Job drawing, mm, ordinate dimensions from the low corner. One solid piece. Coordinates: 2 decimals unless noted, no trailing zeros. Write each loop counter-clockwise with the first axis right and the second up, starting at its lowest first coordinate (ties: lowest second). Pieces come first, ordered by that corner, then holes. Notation, with made-up numbers: (4.5, 22) - (59.5, 22) arc R5 cw to (59.5, 26) - close; hole circle Ø7 at (31, 18.25). An arc over 180 degrees is marked (long way). Use one line per item in the form item = value. Start each with the question number.
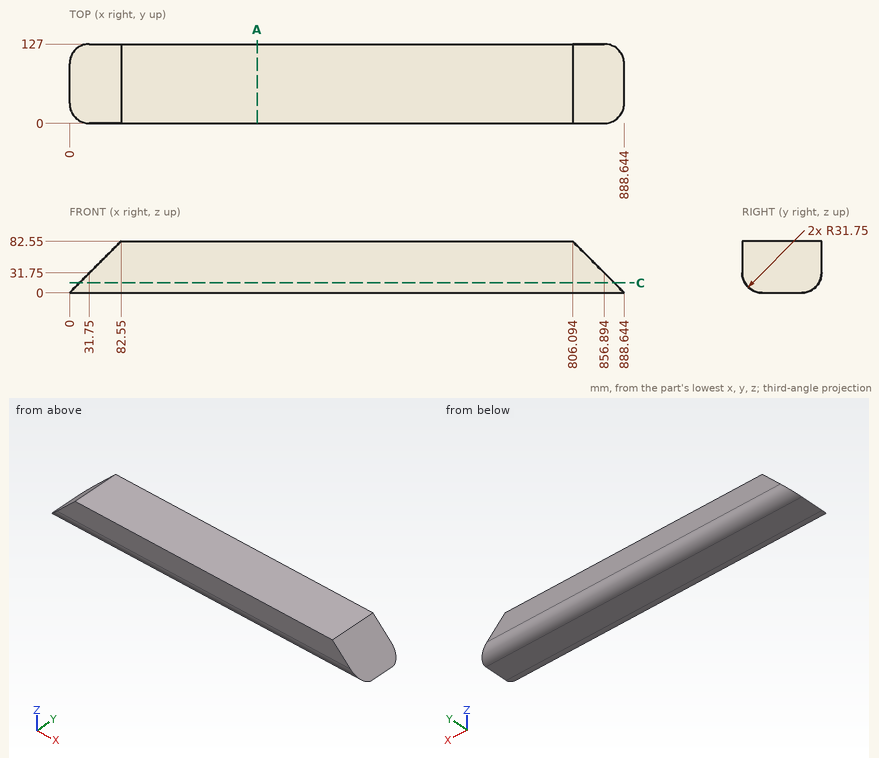
Q1. Drill centre lines: probe 1 along Y at (x, z) = (36, 31); probe 2 along Z at (x, y) = (381, 28.5); probe 3 along Y at (x, z) = (622.5, 11). Where is each one in solid material? Low to high.
Q2. Slice it at A-A (x = 300.5). List the corners of the cut face in (y, z).
Q3. Pin check, flat tips, straight feed: P1, Ø8, axis at x = 471.5, z = 27.5, coming from the +Y side; P2, Ø3, axis at y = 22, z = 40.5, coming from the +X side (1 decimal); P3, Ø2, axis at y = 25.5, z = 67.5, coming from the +X side (1 decimal). Stop position of each tip, or through.
Q4. Slice it at C-C (z = 16). List the corners of the cut face in (x, y) (1 decimal).
Solution:
q1.probe_1 = 0.01 to 126.99
q1.probe_2 = 0.17 to 82.55
q1.probe_3 = 7.72 to 119.28
q2.outline = (0, 31.75) arc R31.75 ccw to (31.75, 0) - (95.25, 0) arc R31.75 ccw to (127, 31.75) - (127, 82.55) - (0, 82.55) - close
q3.P1 = 127
q3.P2 = 849.6
q3.P3 = 822.1
q4.outline = (16, 4.2) - (872.6, 4.2) - (872.6, 122.8) - (16, 122.8) - close
